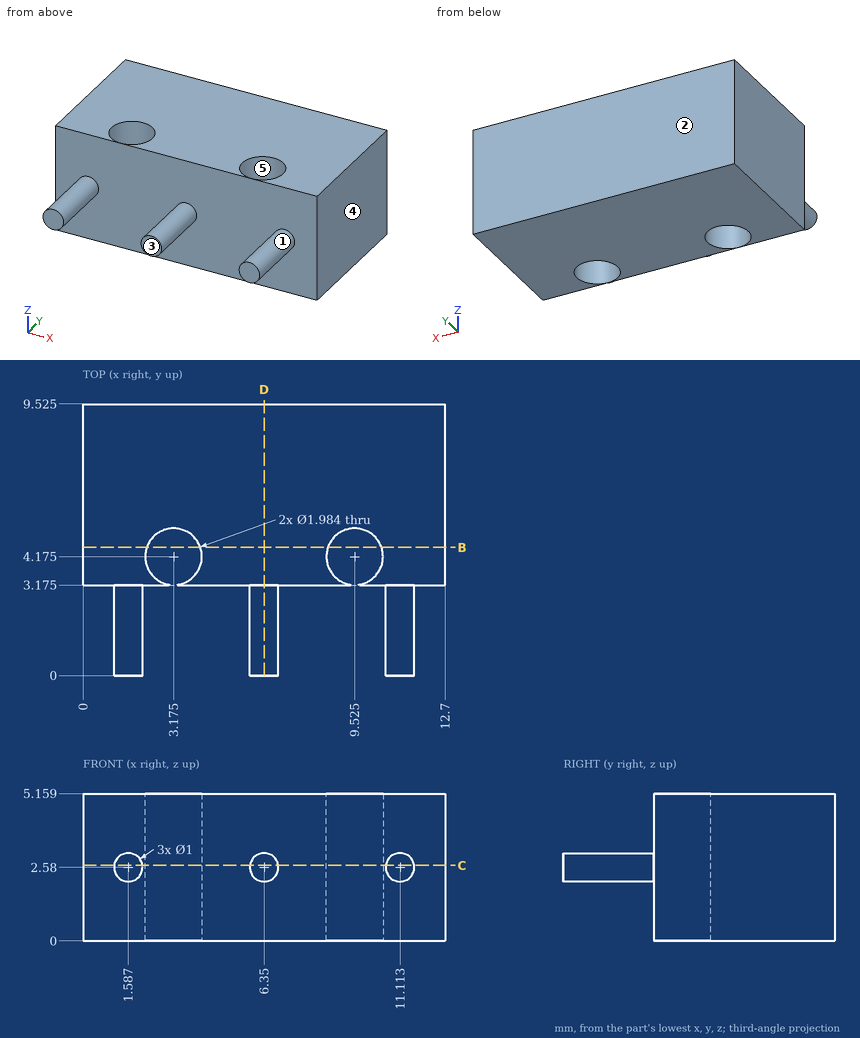
Here's the drawing with two shaded views (mm, measured from the low corner). I have some questions. A direction names the side the tool comes from. Round coordinates to 2 decimals unless told otherwise and drop trailing zeros. Order: outer loops, then holes, each group sorted by start corner. A loop starts at its lowest first (then second) coordinate and runs counter-clockwise, first axis right, second up. Notation, with made-up numbers: (59, 22.25) -> (103, 22.25) arc R33 ccw to (103, 59.25) -> close; hole circle Ø5 at (89.5, -11). An arc over 180 degrees is marked (long way). Use a Markdown table: item, result. Add a question column.
(1) Suppose I cut it at C-C, the plane z = 2.65. Please give me the cut outline in (x, y) (1 decimal).
(2) If we mould it in two halves opening along X, with no side actions, what happens to the marked faces 3, 4 and 5? For each: released by +X, released by -X, zero draft, split by the parting line, or undercut.
(3) Suppose I cut it at B-B, the plane y = 4.5. Please give me the cut outline in (x, z).
(4) For the marked faces 1 and 2, which set-ups out of +Z, -Z, +X, -X, +Y, -Y let a thin tool reach every point of the face, with its end or its side?
(5) I need wall thicknesses on line 1 along X through (y, z) = (4, 3.05); line 2 along X through (y, z) = (4.5, 2.55); line 3 along Y through (x, z) = (5, 4.35) (1 decimal). Which ranges of each line are inside material? Lowest first, please.
(6) Suppose I cut it at D-D, the plane x = 6.35. Please give me the cut outline in (y, z) (1 decimal).
(7) For pin 1 Ø1.2 at (x, y) = (3.175, 4.175) entering from -Z, with a flat end and sliding along its axis, tell me the tip position at first contact or that it passes through.
Verdict:
| question | item | result |
|---|---|---|
| 1 | outline | (0, 3.2) -> (1.1, 3.2) -> (1.1, 0) -> (2.1, 0) -> (2.1, 3.2) -> (5.9, 3.2) -> (5.9, 0) -> (6.8, 0) -> (6.8, 3.2) -> (10.6, 3.2) -> (10.6, 0) -> (11.6, 0) -> (11.6, 3.2) -> (12.7, 3.2) -> (12.7, 9.5) -> (0, 9.5) -> close; hole circle Ø2 at (3.2, 4.2); hole circle Ø2 at (9.5, 4.2) |
| 2 | face 3 | zero draft |
| 2 | face 4 | released by +X |
| 2 | face 5 | undercut |
| 3 | outline | (0, 0) -> (2.24, 0) -> (2.24, 5.16) -> (0, 5.16) -> close; (4.11, 0) -> (8.59, 0) -> (8.59, 5.16) -> (4.11, 5.16) -> close; (10.46, 0) -> (12.7, 0) -> (12.7, 5.16) -> (10.46, 5.16) -> close |
| 4 | face 1 | -Y |
| 4 | face 2 | +Z, -Z, +X, -X, +Y |
| 5 | line 1 | 0 to 2.2, 4.15 to 8.55, 10.5 to 12.7 |
| 5 | line 2 | 0 to 2.24, 4.11 to 8.59, 10.46 to 12.7 |
| 5 | line 3 | 3.2 to 9.5 |
| 6 | outline | (0, 2.1) -> (3.2, 2.1) -> (3.2, 0) -> (9.5, 0) -> (9.5, 5.2) -> (3.2, 5.2) -> (3.2, 3.1) -> (0, 3.1) -> close |
| 7 | pin 1 | through |
